Design review of the part built by this model. Coordinates are the model's own, in mm. Give positions to 0.01 mm unless a question says otherwise; leave off trailing zeros. One line per item, written item: value.
from build123d import *

# Parameters (mm, degrees)
BOSS_EXTRUDE1_DEPTH = 603.25
SKETCH8_R           = 2.565266714
CUT_EXTRUDE4_DEPTH  = 604.996
FILLET1_R           = 2.032
FILLET2_R           = 0.508
SKETCH5_W           = 12.655737404
SKETCH5_H           = 275.477439744
BOSS_EXTRUDE3_DEPTH = 4.572
SKETCH6_R           = 4.617709461
SKETCH6_R_2         = 4.503643825
SKETCH6_R_3         = 4.621904919
SKETCH6_R_4         = 4.672748293
SKETCH6_R_5         = 4.615964847
CUT_EXTRUDE2_DEPTH  = 4.572
SKETCH7_R           = 4.54487388
SKETCH7_R_2         = 4.672668652
CUT_EXTRUDE3_DEPTH  = 4.572
FILLET3_R           = 2.286


with BuildPart() as part:
    # Sketch2 → Boss-Extrude1 (new body)
    with BuildSketch(Plane(origin=(0, 0, 0), x_dir=(1, 0, 0), z_dir=(0, 1, 0))):
        Polygon((-16.258611825, -14.593573265), (-15.211300169, -2.97584616), (-12.901409331, -8.316313776), (2.370242199, 7.164742979), (-1.981461576, 9.939777323), (9.141388175, 10.806426735), (8.274738763, -0.316423015), (5.499704418, 4.03528076), (-9.981352337, -11.236370771), (-4.640884721, -13.546261608), align=None)
        Polygon((-15.391962413, -0.962649654), (-12.616928069, 3.750799497), (2.370242199, -11.236370771), (-2.346798037, -13.546261608), (9.141388175, -14.593573265), (8.094076519, -3.105387053), (5.784185681, -7.822427289), (-9.202984587, 7.164742979), (-4.489535436, 9.939777323), (-16.258611825, 10.806426735), align=None)
    extrude(amount=BOSS_EXTRUDE1_DEPTH)

    # Sketch8 → Cut-Extrude4 (cut)
    with BuildSketch(Plane(origin=(0, 603.25, 0), x_dir=(1, 0, 0), z_dir=(0, 1, 0))):
        with Locations(Location((-3.527048706, -1.915222876, 0), (0, 0, 270))):
            Circle(SKETCH8_R)
    extrude(amount=-CUT_EXTRUDE4_DEPTH, mode=Mode.SUBTRACT)

    # Fillet1
    fillet1_edges = [part.edges().sort_by_distance(p)[0] for p in [
        (9.141388175, 301.625, -10.806426735),
        (9.141388175, 301.625, 14.593573265),
        (-16.258611825, 301.625, 14.593573265),
        (-16.258611825, 301.625, -10.806426735),
    ]]
    fillet(fillet1_edges, radius=FILLET1_R)

    # Fillet2
    fillet2_edges = [part.edges().sort_by_distance(p)[0] for p in [
        (-1.981461576, 301.625, -9.939777323),
        (8.274738763, 301.625, 0.316423015),
        (8.094076519, 301.625, 3.105387053),
        (-2.346798037, 301.625, 13.546261608),
        (-4.640884721, 301.625, 13.546261608),
        (-15.211300169, 301.625, 2.97584616),
        (-15.391962413, 301.625, 0.962649654),
        (-4.489535436, 301.625, -9.939777323),
    ]]
    fillet(fillet2_edges, radius=FILLET2_R)

    # Sketch5 → Boss-Extrude3 (add)
    with BuildSketch(Plane(origin=(-0.781752329, 0, -10.033254025), x_dir=(-0.9969782897972478, 0, 0.07768069047681715), z_dir=(-0.07768069047681715, 0, -0.9969782897972478))):
        with Locations((2.46042797, 432.716085527)):
            Rectangle(SKETCH5_W, SKETCH5_H)
    extrude(amount=BOSS_EXTRUDE3_DEPTH)

    # Sketch6 → Cut-Extrude2 (cut)
    with BuildSketch(Plane(origin=(-1.136908446, 0, -14.591438766), x_dir=(-0.9969782897972478, 0, 0.07768069047681722), z_dir=(-0.07768069047681722, 0, -0.9969782897972478))):
        with Locations((2.46042797, 545.232588529)):
            Circle(SKETCH6_R)
        with Locations((2.46042797, 513.854170907)):
            Circle(SKETCH6_R_2)
        with Locations((2.46042797, 479.255100803)):
            Circle(SKETCH6_R_3)
        with Locations((2.46042797, 446.301604006)):
            Circle(SKETCH6_R_4)
        with Locations((2.46042797, 414.342225806)):
            Circle(SKETCH6_R_5)
    extrude(amount=-CUT_EXTRUDE2_DEPTH, mode=Mode.SUBTRACT)

    # Sketch7 → Cut-Extrude3 (cut)
    with BuildSketch(Plane(origin=(-1.136908446, 0, -14.591438766), x_dir=(-0.9969782897972478, 0, 0.07768069047681712), z_dir=(-0.07768069047681712, 0, -0.9969782897972478))):
        with Locations((2.610241648, 377.377881706)):
            Circle(SKETCH7_R)
        with Locations((2.157369038, 338.135767483)):
            Circle(SKETCH7_R_2)
    extrude(amount=-CUT_EXTRUDE3_DEPTH, mode=Mode.SUBTRACT)

    # Fillet3
    fillet3_edges = [part.edges().sort_by_distance(p)[0] for p in [
        (-0.326311914, 301.625, 1.711929695),
        (-6.767665082, 301.625, 2.09846349),
        (-3.376968255, 301.625, -1.338726647),
        (-3.76350205, 301.625, 5.102626521),
    ]]
    fillet(fillet3_edges, radius=FILLET3_R)


solid = part.part
Item 1: Clearance check with flat-ended pins moving along their axes: P1, Ø5, axis at x = -7.5, y = 135.5, coming from the +Z side; P2, Ø4, axis at x = -5.5, z = -8.5, coming from the -Y side; P3, Ø1.6, axis at x = -4, z = -13, coming from the +Y side; P4, Ø12, axis at x = -9, y = 321.5, coming from the -Z side. State where each tip first meets the part, or that it passes through.
Returned:
P1: z = 14.03
P2: y = 0
P3: y = 570.45
P4: z = -14.45
Item 2: Draft analysis for pull direction X (two halves, no side actions). For faces 1 (the cylindrical face through (-2.82, 549.81, -12.2)), 2 (the flat face through (-3.502, 434.644, -14.407)), 3 (the cylindrical face through (-2.58, 372.94, -12.22)), 4 (the flat face through (-3, 603.25, -1)), state which applies: pulls with the +X half, pulls with the -X half, needs draft (parallel to the pull), parting line crosses it, or undercut.
Returned:
face 1: undercut
face 2: pulls with the -X half
face 3: undercut
face 4: needs draft
Item 3: Add section A-A on y = 403. Count the separate pieces of the cut face and the enclosed holes in it, plus the area to 3 significant figures.
Returned:
separate pieces: 1
enclosed holes: 2
area: 405 mm²
Item 4: To check wall thickness, follow line 1 along Z through (x, y) = (7.25, 210); line 2 along X through (y, z) = (550, 2); line 3 along X through (y, z) = (419, -8.75). State the ranges of each line that lie inside material, in increasing order. Write a range as from..to.
Returned:
line 1: -10.6..-1.29, 4.83..14.35
line 2: -7.71..-6.09, -0.96..0.65
line 3: -16.09..-6.51, -0.12..8.96
